Input: dimensioned drawing with shaded views. Units: mm. Origin: part minimum x, y, z. Give positions to 0.01 mm unless a question says otherwise; leave off trailing zeros. Write each loop counter-clockwise with the first axis right and the second up, starting at its lowest first coordinate (ties: lowest second). Pieces come first, ordered by that corner, then holes. Notation, with made-up numbers: M 18,70 L 28,70 A11 cw 28,74 Z; hole C 44,21 d2. An arc over 180 degrees is marked long. Answer as a JSON object with one key per item and string values.
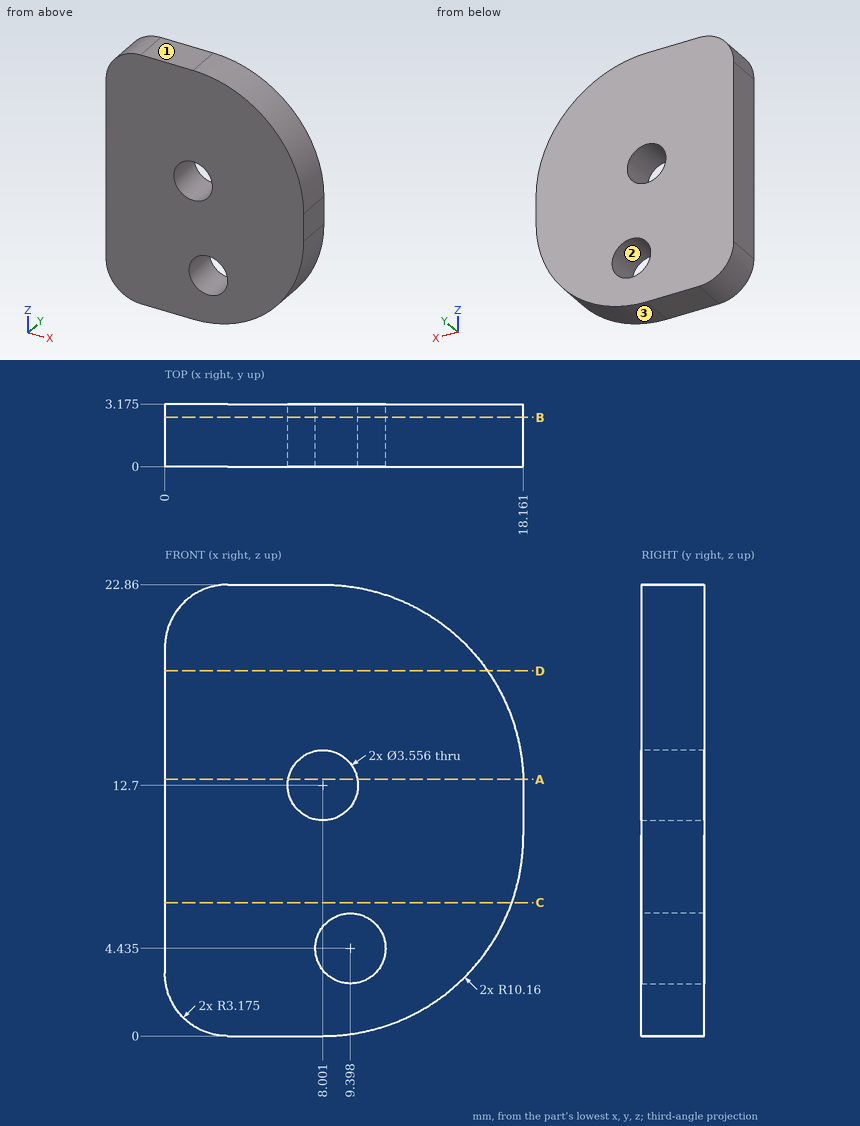
1) Cut plane D-D on z = 18.5. Return loops of the section in (x, y) (1 decimal).
Geometry check:
{"outline": "M 0,0 L 16.3,0 L 16.3,3.2 L 0,3.2 Z"}
2) Cut plane B-B on y = 2.5. Give the number of separate pieces and of enclosed holes in the cut face, and give its area (3 significant figures).
Geometry check:
{"separate pieces": "1", "enclosed holes": "2", "area": "347 mm2"}
3) Cut plane A-A on z = 13. Return loops of the section in (x, y) (1 decimal), and give its area (3 significant figures).
Geometry check:
{"outline": "M 0,0 L 6.2,0 L 6.2,3.2 L 0,3.2 Z; M 9.8,0 L 18.2,0 L 18.2,3.2 L 9.8,3.2 Z", "area": "46.5 mm2"}
4) Pull-direction query (Z, two-part tool) for the marked faces 1, 2 and 3; classes: pulls with the +Z half, pulls with the -Z half, needs draft (parallel to the pull), parting line crosses it, or undercut.
Geometry check:
{"face 1": "pulls with the +Z half", "face 2": "undercut", "face 3": "pulls with the -Z half"}
5) Line query: line 1 (Z direction, x = 7, y = 1.55); line 2 (X direction, y = 0.65, z = 10); line 3 (Z direction, x = 7.5, y = 1.95). Output: solid intervals per line, ascending. Write a range as from..to.
Geometry check:
{"line 1": "z = 0..11.23, 14.17..22.86", "line 2": "x = 0..18.16", "line 3": "z = 0..10.99, 14.41..22.86"}
6) Contact query for a flat-ended pin moving along its axis: P1, Ø1.5, axis at y = 1, z = 4.5, coming from the +X side. Output: stop coordinate, or through.
Geometry check:
{"P1": "stops at x = 16.9"}
7) Cut plane C-C on z = 6.75. Return loops of the section in (x, y) (1 decimal), and give its area (3 significant figures).
Geometry check:
{"outline": "M 0,0 L 17.6,0 L 17.6,3.2 L 0,3.2 Z", "area": "55.8 mm2"}
